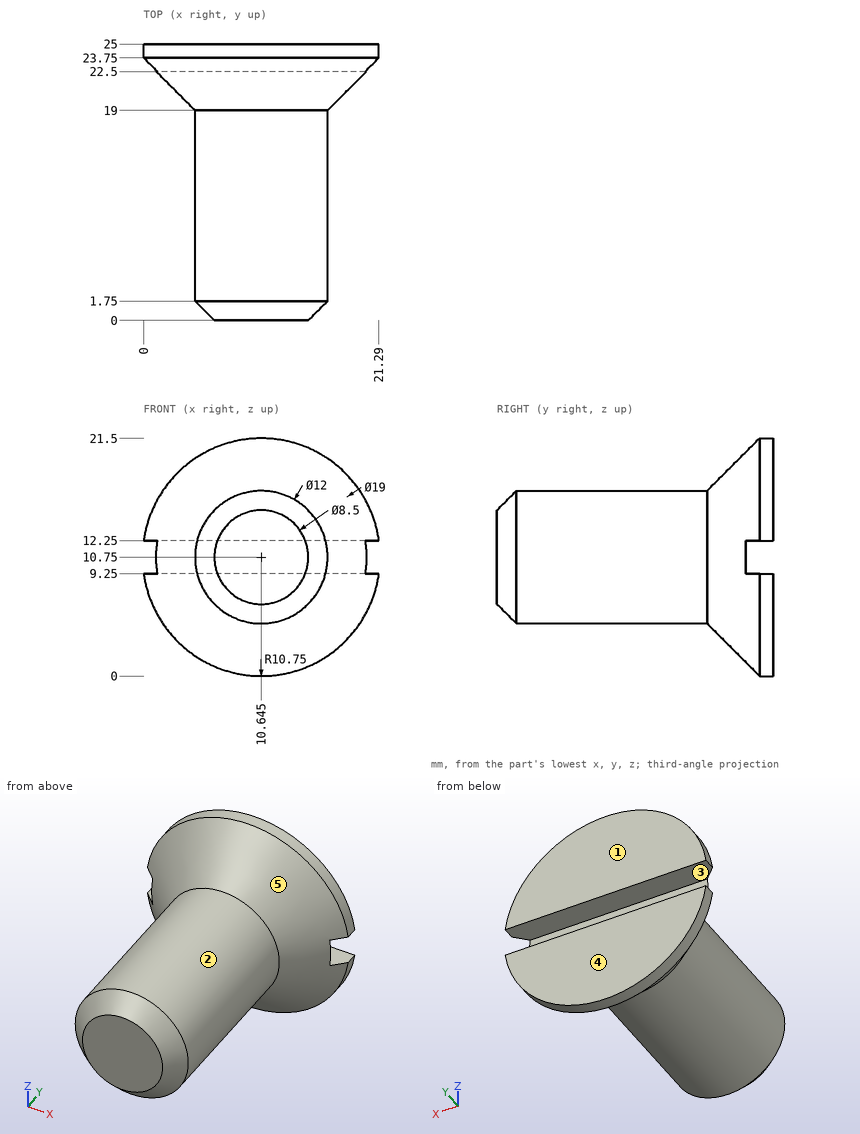
Job drawing, mm, ordinate dimensions from the low corner. One solid piece. A direction names the side the tool comes from. Round coordinates to 2 decimals unless told otherwise and drop trailing zeros. Return JSON: item names as keys, results as strings. Group by question number.
(1) Two-plate mould, pull along Z, no slides. Class the marked faces 3, 4 and 5: +Z half, -Z half, draft (parallel to the pull), parting line (faces both ways), or undercut.
(2) Drill centre lines: probe 1 along Y at (x, z) = (3.5, 11.75) (1 decimal); probe 2 along Y at (x, z) = (6.5, 11.5); probe 3 along Z at (x, y) = (9.25, 3.5) (1 decimal). Where is each one in solid material? Low to high.
(3) Pin check, flat tips, straight feed: pin 1 Ø3 at (y, z) = (12.5, 7.5) entering from -X; pin 2 Ø1.5 at (x, z) = (9.5, 11) entering from +Y; pin 3 Ø0.8 at (x, y) = (12.5, 23.5) entering from +Z; pin 4 Ø3 at (x, z) = (11.5, 15) entering from -Y. Stop position of each tip, or through.
(4) Which spindle directions (+Z, -Z, +X, -X, +Y, -Y) get a long thin tool onto all of the face, cutting with end or side? Do the marked faces 1 and 2. Say none if no direction does.
Returned:
{
 "1": {"face 3": "undercut", "face 4": "draft", "face 5": "parting line"},
 "2": {"probe 1": "20.2 to 22.5", "probe 2": "0 to 22.5", "probe 3": "4.9 to 16.6"},
 "3": {"pin 1": "x = 4.91", "pin 2": "y = 22.5", "pin 3": "z = 21.39", "pin 4": "y = 0"},
 "4": {"face 1": "+Z, -Z, +X, -X, +Y", "face 2": "-Y"}
}
